Build history of the part. All positions in model axes, mm. A direction names the side the tool comes from. Give positions to 0.01 mm unless a question says otherwise; leave off trailing zeros. Order: outer loops, then holes, each group sorted by start corner. A loop starts at its lowest first (then second) coordinate and runs counter-clockwise, first axis right, second up. Notation, with made-up numbers: (5, 46.25) -> (52, 46.25) arc R25 ccw to (52, 58.25) -> close; hole circle Ø9 at (-5.5, -19). An arc over 180 degrees is marked (long way). Write item = value, one per line. Start each with the question number.
from build123d import *

# Parameters (mm, degrees)
BASELINE_BODY_DEPTH          = 7.5
SKETCH3_R                    = 5
CUT_EXTRUDE1_DEPTH           = 159.837149307
SKETCH4_R                    = 25
BOSS_EXTRUDE2_DEPTH          = 15
SKETCH5_R                    = 12
CUT_EXTRUDE2_DEPTH           = 161.947941894
SKETCH6_R                    = 13
CUT_EXTRUDE3_DEPTH           = 9
CUT_EXTRUDE4_START           = -9
SKETCH7_R                    = 13
CUT_EXTRUDE4_DEPTH           = 9
M4_TAPPED_HOLE6_D            = 3.3
M4_TAPPED_HOLE6_DEPTH        = 9
M4_TAPPED_HOLE6_TIP          = 0.991420021
M4_TAPPED_HOLE8_D            = 3.3
M4_TAPPED_HOLE8_DEPTH        = 9
M4_TAPPED_HOLE8_TIP          = 0.991420021
LIGHTENING_WINDOW_DEPTH      = 160.720036314
LIGHTENING_WINDOW_DEPTH_BACK = 160.720036314
SKETCH17_R                   = 18


with BuildPart() as part:
    # Rocker_Profile → Baseline_Body (new, symmetric)
    with BuildSketch(Plane.XY):
        with BuildLine():
            Line((-97.302083333, -24.966068553), (-1.5625, -29.959282264))
            ThreePointArc((-1.5625, -29.959282264), (17.206458335, -24.57514581), (28.686326507, -8.780357142))
            Line((28.686326507, -8.780357142), (52.641312178, 69.483035715))
            ThreePointArc((52.641312178, 69.483035715), (44.023831603, 96.580885487), (15.628732451, 98.088458997))
            Line((15.628732451, 98.088458997), (-109.107307638, 21.288458997))
            ThreePointArc((-109.107307638, 21.288458997), (-120.2235003, -6.182397046), (-97.302083333, -24.966068553))
        make_face()
    extrude(amount=BASELINE_BODY_DEPTH, both=True)

    # Sketch3 → Cut-Extrude1 (cut, through all)
    with BuildSketch(Plane.XY.offset(7.5)):
        with Locations((-96, 0)):
            Circle(SKETCH3_R)
        with Locations((28.736040089, 76.8)):
            Circle(SKETCH3_R)
    extrude(amount=-CUT_EXTRUDE1_DEPTH, mode=Mode.SUBTRACT)

    # Sketch4 → Boss-Extrude2 (add, symmetric)
    with BuildSketch(Plane.XY):
        Circle(SKETCH4_R)
    extrude(amount=BOSS_EXTRUDE2_DEPTH, both=True)

    # Sketch5 → Cut-Extrude2 (cut, through all)
    with BuildSketch(Plane.XY.offset(15)):
        Circle(SKETCH5_R)
    extrude(amount=-CUT_EXTRUDE2_DEPTH, mode=Mode.SUBTRACT)

    # Sketch6 → Cut-Extrude3 (cut)
    with BuildSketch(Plane.XY.offset(15)):
        Circle(SKETCH6_R)
    extrude(amount=-CUT_EXTRUDE3_DEPTH, mode=Mode.SUBTRACT)

    # Sketch7 → Cut-Extrude4 (cut)
    with BuildSketch(Plane(origin=(0, 0, -15), x_dir=(-1, 0, 0), z_dir=(0, 0, -1)).offset(CUT_EXTRUDE4_START)):
        with Locations(Location((0, 0, 0), (0, 0, 180))):
            Circle(SKETCH7_R)
    extrude(amount=CUT_EXTRUDE4_DEPTH, mode=Mode.SUBTRACT)

    # M4 Tapped Hole6
    with Locations(Plane.XY.offset(15)):
        with Locations((-15.588457268, -9), (0, 18), (15.588457268, -9)):
            Hole(M4_TAPPED_HOLE6_D / 2, depth=M4_TAPPED_HOLE6_DEPTH)
            with Locations((0, 0, -(M4_TAPPED_HOLE6_DEPTH + M4_TAPPED_HOLE6_TIP / 2))):  # 118° drill point
                Cone(0, M4_TAPPED_HOLE6_D / 2, M4_TAPPED_HOLE6_TIP, mode=Mode.SUBTRACT)

    # M4 Tapped Hole8
    with Locations(Plane(origin=(0, 0, -15), x_dir=(-1, 0, 0), z_dir=(0, 0, -1))):
        with Locations((-15.588457268, -9), (0, 18), (15.585467422, -8.998273811)):
            Hole(M4_TAPPED_HOLE8_D / 2, depth=M4_TAPPED_HOLE8_DEPTH)
            with Locations((0, 0, -(M4_TAPPED_HOLE8_DEPTH + M4_TAPPED_HOLE8_TIP / 2))):  # 118° drill point
                Cone(0, M4_TAPPED_HOLE8_D / 2, M4_TAPPED_HOLE8_TIP, mode=Mode.SUBTRACT)

    # Sketch17 → Lightening_Window (cut, two sides: drawn at the far end of the back side and taken through both)
    with BuildSketch(Plane.XY.offset(7.5).offset(-LIGHTENING_WINDOW_DEPTH_BACK)):
        with Locations((-40, 30)):
            Circle(SKETCH17_R)
    extrude(amount=LIGHTENING_WINDOW_DEPTH + LIGHTENING_WINDOW_DEPTH_BACK, mode=Mode.SUBTRACT)


solid = part.part
(1) Cut at A-A, the plane y = 30. Give the cut face in (x, z).
(2) Cut at C-C, the plane x = -40. Give the cut face in (y, z), plus the area to 3 significant figures.
(3) Mould opens along Y. For faces 4 (the face through (-15, 37, -7.5)), 5 (the face through (-50.102, -27.428, 0.105)), 6 (the face through (-11.99, 0.53, 0.08)) say: released by +Y, released by -Y, zero draft, split by the parting line, or undercut.
(4) 3-axis set-ups, long thin cutter, end or side, ignore diameter. For faces 1 (the face through (9, 9, -6)), 2 (the face through (9, -9, 6)), 3 (the face through (-120.33, -5.75, 0.11)): which of +Z, -Z, +X, -X, +Y, -Y reach the whole face in a straight line?
(5) Wall check: line 1 (Y direction, x = 0, z = 12); line 2 (Z direction, x = -89.5, y = 29.5); line 3 (X direction, y = -9, z = 8.5). Give the ranges that are in metal, low to high. Write a range as [from, to].
(6) Cut at B-B, the plane x = 4. Give the cut face in (y, z), plus the area to 3 significant figures.
(7) Flat gauge pins, fed straight in: P1, Ø2.5, axis at x = 0, y = 18, coming from the -Z side; P2, Ø6, axis at x = 26.5, y = 43.5, coming from the +Z side; P3, Ø3, axis at y = 69, z = 0, coming from the +X side. Where does each tip first touch, or does it go through?
(8) Cut at D-D, the plane y = -16.5. Give the cut face in (x, z).
Results:
q1.outline = (-94.96, -7.5) -> (-58, -7.5) -> (-58, 7.5) -> (-94.96, 7.5) -> close; (-22, -7.5) -> (40.56, -7.5) -> (40.56, 7.5) -> (-22, 7.5) -> close
q2.outline = (-27.95, -7.5) -> (12, -7.5) -> (12, 7.5) -> (-27.95, 7.5) -> close; (48, -7.5) -> (63.84, -7.5) -> (63.84, 7.5) -> (48, 7.5) -> close
q2.area = 837 mm2
q3.face_4 = zero draft
q3.face_5 = released by -Y
q3.face_6 = undercut
q4.face_1 = -Z
q4.face_2 = +Z
q4.face_3 = +Z, -Z, -X
q5.line_1 = [-25, -13], [13, 16.35], [19.65, 25]
q5.line_2 = [-7.5, 7.5]
q5.line_3 = [-23.32, -17.24], [-13.94, -9.38], [9.38, 13.94], [17.24, 23.32]
q6.outline = (-29.73, -7.5) -> (-24.68, -7.5) -> (-24.68, -15) -> (-12.37, -15) -> (-12.37, -6) -> (-11.31, -6) -> (-11.31, 6) -> (-12.37, 6) -> (-12.37, 15) -> (-24.68, 15) -> (-24.68, 7.5) -> (-29.73, 7.5) -> close; (11.31, -6) -> (12.37, -6) -> (12.37, -15) -> (24.68, -15) -> (24.68, -7.5) -> (90.93, -7.5) -> (90.93, 7.5) -> (24.68, 7.5) -> (24.68, 15) -> (12.37, 15) -> (12.37, 6) -> (11.31, 6) -> close
q6.area = 1,830 mm2
q7.P1 = -5.76
q7.P2 = 7.5
q7.P3 = 52.93
q8.outline = (-114.78, -7.5) -> (-18.78, -7.5) -> (-18.78, -15) -> (18.78, -15) -> (18.78, -7.5) -> (25.05, -7.5) -> (25.05, 7.5) -> (18.78, 7.5) -> (18.78, 15) -> (-18.78, 15) -> (-18.78, 7.5) -> (-114.78, 7.5) -> close
